Design review of the part built by this model. Coordinates are the model's own, in mm. Coordinates: 2 decimals unless noted, no trailing zeros. Write each loop counter-clockwise with the first axis right and the second up, starting at its lowest first coordinate (ties: lowest second). Pieces come first, ordered by that corner, then holes.
Q1. To check wall thickness, follow probe 1 along Y at (x, z) = (-4, 3.6); probe 2 along Z at (x, y) = (-3.75, 2); probe 3 along Y at (x, z) = (-0.5, 4.2). State the ranges of each line that lie inside material, in increasing order.
Q2. Add section A-A, the plane x = -1.75. Give the boundary of the cut face in (y, z), plus the area to 3 significant figures.
Q3. Add section B-B, the plane z = 4.2. Give the boundary of the cut face in (x, y), plus the area to 3 significant figures.
Q4. Add section C-C, the plane y = 1.25. Give the boundary of the cut face in (x, z), plus the area to 3 significant figures.
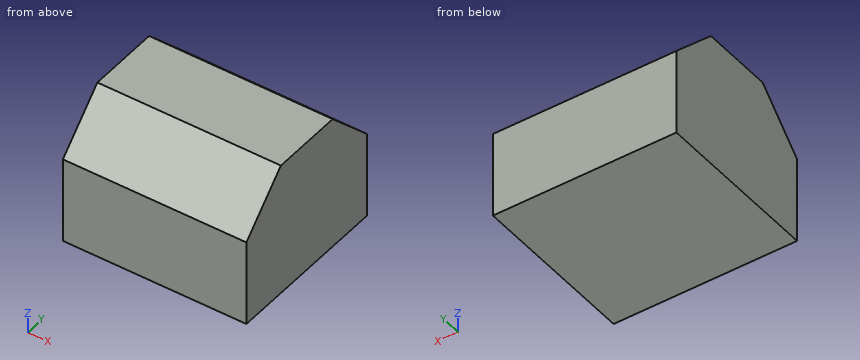
from build123d import *

# Parameters (mm, degrees)
SKETCH_1_W      = 6.8
SKETCH_1_H      = 6.3
EXTRUDE_1_DEPTH = 5
CHAMFER_1_SIZE  = 1.8


with BuildPart() as part:
    # 草图1 → 凸台-拉伸1 (new body)
    with BuildSketch(Plane.XY):
        with Locations((-2.131657577, -0.555911138)):
            Rectangle(SKETCH_1_W, SKETCH_1_H)
    extrude(amount=EXTRUDE_1_DEPTH)

    # 倒角1
    chamfer_1_edges = [part.edges().sort_by_distance(p)[0] for p in [
        (-2.131657577, 2.594088862, 5),
        (-2.131657577, -3.705911138, 5),
    ]]
    chamfer(chamfer_1_edges, length=CHAMFER_1_SIZE)


solid = part.part
Here are the results:
1. probe 1: y = -3.31 to 2.19
1. probe 2: z = 0 to 3.79
1. probe 3: y = -2.71 to 1.59
2. outline: (-3.71, 0) - (2.59, 0) - (2.59, 3.2) - (0.79, 5) - (-1.91, 5) - (-3.71, 3.2) - close
2. area: 28.3 mm2
3. outline: (-5.53, -2.71) - (1.27, -2.71) - (1.27, 1.59) - (-5.53, 1.59) - close
3. area: 29.2 mm2
4. outline: (-5.53, 0) - (1.27, 0) - (1.27, 4.54) - (-5.53, 4.54) - close
4. area: 30.9 mm2
